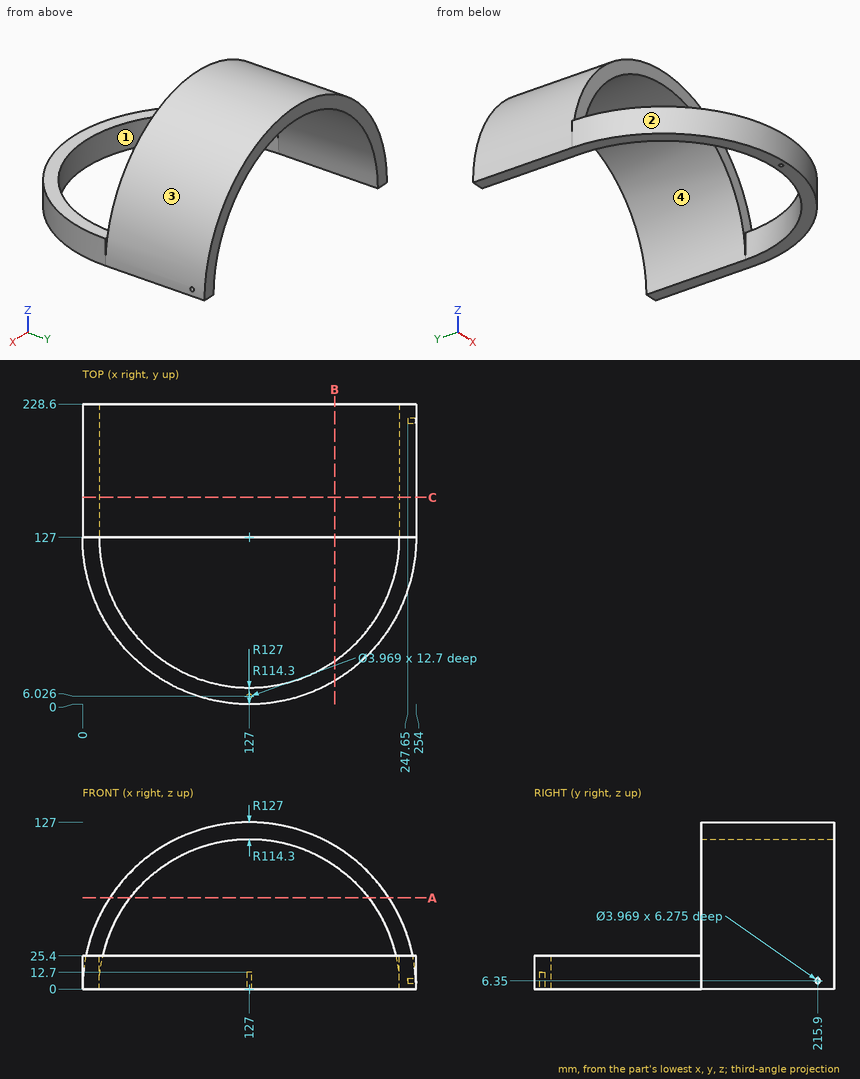
Study the drawing (mm; zero at the part's minimum x, y, z) and answer. A direction names the side the tool comes from. Give positions to 0.01 mm unless a question says otherwise; leave off trailing zeros. Write each loop counter-clockwise with the first axis right and the second up, starting at its lowest first coordinate (ties: lowest second). Pieces come first, ordered by that corner, then holes. Notation, with made-up numbers: (17, 5) - (49, 5) arc R25 ccw to (49, 41) - close; hole circle Ø3 at (-26, 36). An arc over 180 degrees is marked (long way). Write item = value, one per line. Start each with the question number.
Item 1: Find section C-C (y = 157.5). Give the vertices of the cut face in (x, z).
Item 2: A tool of negligible diameter and unlimited length cuts with its end or side. For the marked faces 3 and 4, from which of +Z, -Z, +X, -X, +Y, -Y can it reach the whole face along a straight path? Write none if from no direction.
Item 3: The mould has two halves that part along X. Classify the marked faces 1 and 2: +X half, -X half, draft (parallel to the pull), parting line (faces both ways), or undercut.
Item 4: Find section A-A (z = 69.5). Give the vertices of the cut face in (x, y) (1 decimal), then the cut area to 3 significant figures.
Item 5: Each of these flat-tipped pins is pushed along its axis until it touches: P1, Ø1.5, axis at x = 90.5, y = 187.5, coming from the +Z side (1 decimal); P2, Ø4, axis at y = 175, z = 77.5, coming from the -X side; P3, Ø6.5, axis at x = 127, y = 6.03, coming from the +Z side. Where does it stop, or does it pass through?
Item 6: Find the intervals of material crossed by probe 1 along Y at (x, z) = (75, 107); probe 2 along X at (y, z) = (30.5, 7) (1 decimal); probe 3 along Y at (x, z) = (127, 4.75), in increasing order. Write a range as [from, to].
Item 7: Find section B-B (x = 192). Give the vertices of the cut face in (y, z) (1 decimal), then the cut area to 3 significant figures.
Response:
q1.outline = (0, 0) - (12.7, 0) arc R114.3 cw to (241.3, 0) - (254, 0) arc R127 ccw to start
q2.face_3 = +Z, +Y
q2.face_4 = -Z, +Y
q3.face_1 = undercut
q3.face_2 = parting line
q4.outline = (20.7, 127) - (36.3, 127) - (36.3, 228.6) - (20.7, 228.6) - close; (217.7, 127) - (233.3, 127) - (233.3, 228.6) - (217.7, 228.6) - close
q4.area = 3,160 mm²
q5.P1 = 121.9
q5.P2 = 24.88
q5.P3 = 25.4
q6.probe_1 = [127, 228.6]
q6.probe_2 = [44.4, 65.7], [188.3, 209.6]
q6.probe_3 = [0, 4.04], [8.01, 12.7]
q7.outline = (17.9, 0) - (33, 0) - (33, 25.4) - (17.9, 25.4) - close; (127, 94) - (228.6, 94) - (228.6, 109.1) - (127, 109.1) - close
q7.area = 1,920 mm²
